Check sheet for the modelled part. Datum: model origin and axes. Units: mm. Face numbers are marked on the shaded views. Coordinates: 2 decimals unless noted, no trailing zeros. Write each loop counter-clockwise with the first axis right and the second up, starting at its lowest first coordinate (ties: lowest second). Pieces come first, ordered by that corner, then holes. Notation, with made-up numbers: (52, 70) - (105, 70) arc R25 ccw to (105, 97) - close; hole circle Ø6 at (19.5, -23.5). An arc over 180 degrees is marked (long way). Use one line per item in the form item = value. Start each with the question number.
1. Go/stop test with flat-tipped pins: pin 1 Ø5 at (x, z) = (2.5, 0) entering from +Y; pin 2 Ø2 at (x, y) = (-1.5, 14.5) entering from +Z; pin 3 Ø2 at (y, z) = (40.5, -12) entering from +X. Record where each tip stops, or that it passes through.
2. Draft check along Y on the marked faces 1, 2 and 3. Enter one of: +Y half, -Y half, draft (parallel to the pull), parting line (faces both ways), or undercut.
3. Cross-section at A-A on x = 0. Give the number of separate pieces and of enclosed holes in the cut face, then the cut area to 3 significant figures.
4. Scan lines: line 1 along X through (y, z) = (1.15, 0); line 2 along Z through (x, y) = (0, 43.1); line 3 along Y through (x, z) = (6, -4). Record each from-to range of solid material in increasing order.
5. Cross-section at C-C on y = 3. Record the boundary of the cut face in (x, z), then the cut area to 3 significant figures.
6. Cross-section at D-D on x = -7. Record the boundary of the cut face in (y, z), then the cut area to 3 significant figures.
```python
from build123d import *

# Parameters (mm, degrees)
SKETCH1_R           = 4
BOSS_EXTRUDE1_DEPTH = 45.15
SKETCH2_W           = 40
SKETCH2_H           = 37.65
CUT_EXTRUDE1_DEPTH  = 26
SKETCH3_R           = 1.65
CUT_EXTRUDE2_DEPTH  = 46.15
CIRPATTERN1_COUNT   = 4
FILLET1_R           = 2
CUT_EXTRUDE4_DEPTH  = 37.65


with BuildPart() as part:
    # Sketch1 → Boss-Extrude1 (new body)
    with BuildSketch(Plane(origin=(0, 0, 0), x_dir=(1, 0, 0), z_dir=(0, 1, 0))):
        with BuildLine():
            Line((-12.5, 15), (-12.5, 20))
            Line((-12.5, 20), (12.5, 20))
            Line((12.5, 20), (12.5, 15))
            Line((12.5, 15), (9.367496998, 7.5))
            ThreePointArc((9.367496998, 7.5), (0, -12), (-9.367496998, 7.5))
            Line((-9.367496998, 7.5), (-12.5, 15))
        make_face()
        Circle(SKETCH1_R, mode=Mode.SUBTRACT)
    extrude(amount=BOSS_EXTRUDE1_DEPTH)

    # Sketch2 → Cut-Extrude1 (cut, through all)
    with BuildSketch(Plane.ZY.offset(12.5)):
        with Locations((5, 22.575)):
            Rectangle(SKETCH2_W, SKETCH2_H)
    extrude(amount=-CUT_EXTRUDE1_DEPTH, mode=Mode.SUBTRACT)

    # Sketch3 → Cut-Extrude2 (cut, through all)
    with BuildSketch(Plane(origin=(0, 45.15, 0), x_dir=(1, 0, 0), z_dir=(0, 1, 0))):
        with Locations((0, 7)):
            Circle(SKETCH3_R)
    cut_extrude2 = extrude(amount=-CUT_EXTRUDE2_DEPTH, mode=Mode.SUBTRACT)

    # CirPattern1: Cut-Extrude2 ×4 about axis
    cirpattern1_axis = Axis((0, 0, 0), (0, 1, 0))
    for i in range(1, CIRPATTERN1_COUNT):
        add(cut_extrude2.rotate(cirpattern1_axis, i * 360 / CIRPATTERN1_COUNT), mode=Mode.SUBTRACT)

    # Fillet1
    fillet1_edges = [part.edges().sort_by_distance(p)[0] for p in [
        (9.367496998, 43.275, -7.5),
        (-9.367496998, 43.275, -7.5),
        (9.367496998, 1.875, -7.5),
        (-9.367496998, 1.875, -7.5),
    ]]
    fillet(fillet1_edges, radius=FILLET1_R)

    # Sketch4 → Cut-Extrude4 (cut)
    with BuildSketch(Plane(origin=(0, 3.75, 0), x_dir=(1, 0, 0), z_dir=(0, 1, 0))):
        with BuildLine():
            Line((-12.5, 15), (12.5, 15))
            ThreePointArc((12.5, 15), (0, 19.52562419), (-12.5, 15))
        make_face()
    extrude(amount=CUT_EXTRUDE4_DEPTH, mode=Mode.SUBTRACT)


solid = part.part
```
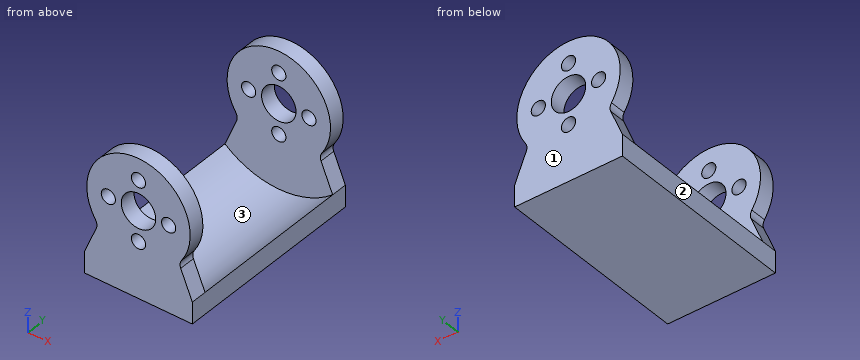
Final values:
q1.pin_1 = 45.15
q1.pin_2 = -19.36
q1.pin_3 = 11.43
q2.face_1 = +Y half
q2.face_2 = draft
q2.face_3 = undercut
q3.separate_pieces = 7
q3.enclosed_holes = 0
q3.area = 148 mm²
q4.line_1 = -12 to -8.65, -5.35 to -4, 4 to 5.35, 8.65 to 12
q4.line_2 = -20 to -8.65, -5.35 to -4, 4 to 5.35, 8.65 to 12
q4.line_3 = 0 to 3.75, 41.4 to 45.15
q5.outline = (-12.5, -20) - (12.5, -20) - (12.5, -15) - (9.8, -8.54) arc R2 cw to (9.98, -6.66) arc R12 ccw (long way) to (-9.98, -6.66) arc R2 cw to (-9.8, -8.54) - (-12.5, -15) - close; hole circle Ø3.3 at (-7, 0); hole circle Ø8 at (0, 0); hole circle Ø3.3 at (0, -7); hole circle Ø3.3 at (0, 7); hole circle Ø3.3 at (7, 0)
q5.area = 599 mm²
q6.outline = (0, -20) - (45.15, -20) - (45.15, -1.65) - (41.4, -1.65) - (41.4, -18.23) - (3.75, -18.23) - (3.75, -1.65) - (0, -1.65) - close; (0, 1.65) - (3.75, 1.65) - (3.75, 9.75) - (0, 9.75) - close; (41.4, 1.65) - (45.15, 1.65) - (45.15, 9.75) - (41.4, 9.75) - close
q6.area = 265 mm²
